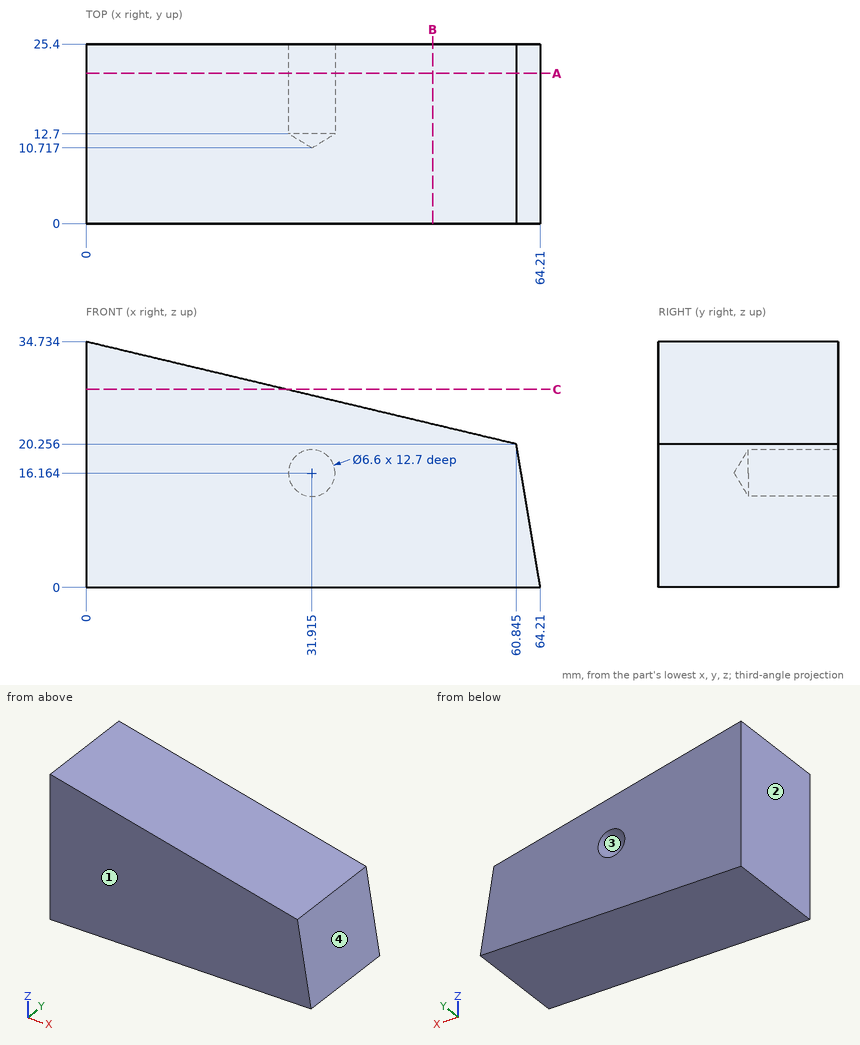
Geometry check sheet. Reference: drawing and pictorial views, mm from the part's lowest x, y, z. Give positions to 0.01 mm unless a question says otherwise; leave off trailing zeros. Order: outer loops, then holes, each group sorted by start corner. A loop starts at its lowest first (then second) coordinate and runs counter-clockwise, first axis right, second up. Notation, with made-up numbers: M 33,65.25 L 60,65.25 A18 ccw 60,96.25 Z; hole C -14,28 d6. An arc over 180 degrees is marked long. Use one line per item in the form item = value. Start each with the question number.
Q1. Go/stop test with flat-tipped pins: pin 1 Ø4 at (x, y) = (51, 13) entering from +Z; pin 2 Ø5.5 at (x, z) = (31.92, 16.16) entering from +Y. Record where each tip stops, or that it passes through.
Q2. Section check B-B (x = 49). Enter the section's corners in (y, z).
Q3. Section check C-C (z = 28). Enter the section's corners in (x, y).
Q4. Scan lines: line 1 along X through (y, z) = (15.25, 19) (1 decimal); line 2 along Z through (x, y) = (31, 22.5) (1 decimal); line 3 along X through (y, z) = (16.75, 16). Record each from-to range of solid material in increasing order. Write a range as [from, to].
Q5. Section check A-A (y = 21.25). Enter the section's corners in (x, z) (1 decimal), then the cut area to 3 significant figures.
Q6. Mould release check, pull along X, two halves, no side actions. Record for the marked faces 1, 2, 3 and 4: +X half, -X half, draft (parallel to the pull), parting line (faces both ways), or undercut.
Evaluation:
q1.pin_1 = 23.07
q1.pin_2 = 12.37
q2.outline = M 0,0 L 25.4,0 L 25.4,23.07 L 0,23.07 Z
q3.outline = M 0,0 L 28.3,0 L 28.3,25.4 L 0,25.4 Z
q4.line_1 = [0, 30.2], [33.6, 61.1]
q4.line_2 = [0, 13], [19.3, 27.4]
q4.line_3 = [0, 28.62], [35.21, 61.55]
q5.outline = M 0,0 L 64.2,0 L 60.8,20.3 L 0,34.7 Z; hole C 31.9,16.2 d6.6
q5.area = 1,670 mm2
q6.face_1 = draft
q6.face_2 = -X half
q6.face_3 = undercut
q6.face_4 = +X half
